from build123d import *

# Parameters (mm, degrees)
SALIENTE_EXTRUIR1_DEPTH = 30


with BuildPart() as part:
    # Croquis1 → Saliente-Extruir1 (new body)
    with BuildSketch(Plane(origin=(0, 0, 0), x_dir=(1, 0, 0), z_dir=(0, 1, 0))):
        with BuildLine():
            ThreePointArc((5.093864637, 5.504774569), (0, 7.5), (-5.093864637, 5.504774569))
            ThreePointArc((-5.093864637, 5.504774569), (-7.629622361, 4.56075577), (-10.095654419, 5.674274793))
            ThreePointArc((-10.095654419, 5.674274793), (-22.5, 0), (-10.095654419, -5.674274793))
            ThreePointArc((-10.095654419, -5.674274793), (-7.629622361, -4.56075577), (-5.093864637, -5.504774569))
            ThreePointArc((-5.093864637, -5.504774569), (0, -7.5), (5.093864637, -5.504774569))
            ThreePointArc((5.093864637, -5.504774569), (7.629622361, -4.56075577), (10.095654419, -5.674274793))
            ThreePointArc((10.095654419, -5.674274793), (22.5, 0), (10.095654419, 5.674274793))
            ThreePointArc((10.095654419, 5.674274793), (7.629622361, 4.56075577), (5.093864637, 5.504774569))
        make_face()
    extrude(amount=SALIENTE_EXTRUIR1_DEPTH)


solid = part.part
Model file for the job. Use its own axes, mm. Round coordinates to 2 decimals unless told otherwise and drop trailing zeros. Order: outer loops, then holes, each group sorted by start corner. A loop starts at its lowest first (then second) coordinate and runs counter-clockwise, first axis right, second up.
(1) Pull direction X, two halves, no side cores. Call faces 1 (the face through (0, 30, 0)), 2 (the face through (22.496, 14.79, 0.24)), 3 (the face through (0.1, 14.8, -7.5)): released by +X, released by -X, zero draft, split by the parting line, or undercut.
(2) Band-saw the part on C-C (z = -2.25). List the corners of the cut face in (x, y), then the cut area to 3 significant figures.
(3) Band-saw the part on A-A (z = 6.25). List the corners of the cut face in (x, y).
(4) Band-saw the part on B-B (y = 14). List the corners of the cut face in (x, z), then the cut area to 3 significant figures.
(5) Pin check, flat tips, straight feed: pin 1 (8 mm diameter, centred on y = 7, z = -4.5, fed in from -X); pin 2 (1 mm diameter, centred on x = -9.5, y = 14.5, fed in from +Z); pin 3 (3 mm diameter, centred on y = 12, z = 4, fed in from -X). Stop position of each tip, or through.
(6) Band-saw the part on D-D (x = 13). List the corners of the cut face in (y, z).
(7) Drill centre lines: line 1 (X direction, y = 9.5, z = 6.75); line 2 (X direction, y = 28, z = -5.25); line 3 (Z direction, x = -7.5, y = 25). Where is each one in solid material? Low to high.
Verdict:
1. face 1: zero draft
1. face 2: undercut
1. face 3: undercut
2. outline: (-22.15, 0) - (22.15, 0) - (22.15, 30) - (-22.15, 30) - close
2. area: 1,330 mm2
3. outline: (-19.15, 0) - (-10.85, 0) - (-10.85, 30) - (-19.15, 30) - close; (-4.15, 0) - (4.15, 0) - (4.15, 30) - (-4.15, 30) - close; (10.85, 0) - (19.15, 0) - (19.15, 30) - (10.85, 30) - close
4. outline: (-10.1, -5.67) arc R3.56 cw to (-5.09, -5.5) arc R7.5 ccw to (5.09, -5.5) arc R3.56 cw to (10.1, -5.67) arc R7.5 ccw (long way) to (10.1, 5.67) arc R3.56 cw to (5.09, 5.5) arc R7.5 ccw to (-5.09, 5.5) arc R3.56 cw to (-10.1, 5.67) arc R7.5 ccw (long way) to start
4. area: 550 mm2
5. pin 1: stops at x = -22.48
5. pin 2: stops at z = 5.58
5. pin 3: stops at x = -22.07
6. outline: (0, -7.23) - (30, -7.23) - (30, 7.23) - (0, 7.23) - close
7. line 1: x = -18.27 to -11.73, -3.27 to 3.27, 11.73 to 18.27
7. line 2: x = -20.36 to -9.62, -5.4 to 5.4, 9.62 to 20.36
7. line 3: z = -4.56 to 4.56
